```python
from build123d import *

# Parameters (mm, degrees)
F0_R     = 1.5
F3_DEPTH = 12.7
F4_DEPTH = 50.8


with BuildPart() as f2:
    # F2: sweep along a path in F1
    with BuildLine(Plane.YZ) as f2_path:
        Line((0, 0), (0.6976816626, 0))
        ThreePointArc((0.6976816626, 0), (3.5907533681, 0.7435624129), (5.7667652809, 2.7899546311))
        Line((5.7667652809, 2.7899546311), (9.0660760179, 8))
    # F0 (on Front) → F2 (sweep)
    with BuildSketch(Plane.XZ):
        Circle(F0_R)
    sweep(path=f2_path.line)

    # F0 (on Front) → F3 (join)
    with BuildSketch(Plane.XZ):
        Circle(F0_R)
    extrude(amount=F3_DEPTH)

    # F4 (add): a face of the model
    f4_faces = [f2.faces().sort_by_distance(p)[0] for p in [
        (0, 9.0660760179, 8),
    ]]
    extrude(f4_faces, amount=F4_DEPTH)


solid = f2.part
```
Input: part model. Units: mm. Frame: model coordinates. A direction names the side the tool comes from. Round coordinates to 2 decimals unless told otherwise and drop trailing zeros. Loops run counter-clockwise (first coordinate to the right, second up) from the corner with the lowest first, then second, coordinate; pieces in that order, holes last. Notation, with made-up numbers: (74, -34) - (120, -34) arc R18 ccw to (120, -1) - close; hole circle Ø2 at (86, 86). An arc over 180 degrees is marked (long way). One line per item, written item: value. Start each with the question number.
(1) Section A-A, the plane x = 0. Return loops of the section in (y, z), plus the area to 3 significant figures.
(2) Access query for faces 1 (the cylindrical face through (0.81, 21.86, 25.84)), 2 (the cylindrical face through (-1.5, -5.91, -0.07)). Directions: +Z, -Z, +X, -X, +Y, -Y. A direction counts if a zero-diameter tool reaches every point of the face in a straight line with its end or side. Return the directions, or none.
(3) Contact query for flat-ended pins moving along their axis: P1, Ø3, axis at y = -6, z = 4.5, coming from the -X side; P2, Ø1, axis at x = 0, y = 18, coming from the -Z side. Output: stop coordinate, or through.
(4) Ray query, line 1 (Y direction, x = -0.8, z = 8); line 2 (Z direction, x = 0.15, y = 20.5); line 3 (X direction, y = 13, z = 16). Return the intervals inside material, ascending. Write a range as [from, to].
Results below:
1. outline: (-12.7, -1.5) - (0.7, -1.5) arc R7.5 ccw to (7.03, 1.99) - (37.51, 50.12) - (34.98, 51.72) - (4.5, 3.59) arc R4.5 cw to (0.7, 1.5) - (-12.7, 1.5) - close
1. area: 229 mm^2
2. face 1: none
2. face 2: -Y
3. P1: through
3. P2: z = 18.51
4. line 1: [7.56, 10.57]
4. line 2: [23.27, 28.85]
4. line 3: [-1.16, 1.16]
